Here's how the part is built. I have some questions about the finished solid (model axes, mm). A direction names the side the tool comes from. Round coordinates to 2 decimals unless told otherwise and drop trailing zeros. Write each loop counter-clockwise with the first axis right and the second up, starting at its lowest first coordinate (ties: lowest second). Pieces come first, ordered by that corner, then holes. Notation, with made-up numbers: (87.25, -5.75) -> (142.25, -5.75) arc R17 ccw to (142.25, 10.25) -> close; hole circle Ø11 at (2.5, 66.25). An arc over 180 degrees is marked (long way). Put each result on its own line as item: value. Start each with the question number.
1) Will these pins go through, and if not, where does the flat tip stop? P1, Ø18.5, axis at x = 944, y = 37, coming from the -Z side (3 decimals); P2, Ø8, axis at x = 1001.5, y = -37, coming from the -Z side (3 decimals); P3, Ø16, axis at y = -16.5, z = 1330, coming from the -X side.
2) I want a section at A-A, the plane z = 1916.5. Give the number of separate pieces and of enclosed holes in the cut face, then the cut area to 3 significant figures.
3) If I drill on line 1 along X through (y, z) = (21.5, 1035.5) (3 decimals); line 2 along X through (y, z) = (-31, 1517) (3 decimals); line 3 along Z through (x, y) = (233, 15.5) (3 decimals), over which ranges is the centre line in solid material (lowest first)? Write a range as [from, to].
4) We'd pull the mould along X, two halves only. Please class faces 1 (the flat face through (28, 3.175, 1032)), 2 (the flat face through (25, 65.088, 1041)), 3 (the flat face through (1570.831, 6, 1022)), 4 (the flat face through (31.75, 34, 1006)): released by +X, released by -X, zero draft, split by the parting line, or undercut.
5) I want a section at B-B, the plane x = 1331.5. List the corners of the cut face in (y, z) for me (1 decimal).
6) Which directions (+Z, -Z, +X, -X, +Y, -Y) give clear straight access to the entire face, cutting with the end or side of a thin tool? Please do faces 5 (the flat face through (607, -50.8, 1041)), 6 (the flat face through (1086, 34, 2041.525)), 7 (the flat face through (1085, -23, 2054.225)).
from build123d import *

# Parameters (mm, degrees)
F3_DEPTH      = 61.9125
F5_DEPTH      = 50.8
F5_DEPTH_BACK = 3.175


with BuildPart() as f3:
    # F2 (on offset) → F3 (new body)
    with BuildSketch(Plane.XZ.offset(-3.175)):
        Polygon((0, 2054.225), (0, 0), (19.05, 0), (31.75, 0), (31.75, 2041.525), (581.025, 2041.525), (581.025, 0), (593.725, 0), (612.775, 0), (631.825, 0), (644.525, 0), (644.525, 2041.525), (1539.08125, 2041.525), (1539.08125, 0), (1551.78125, 0), (1570.83125, 0), (1570.83125, 2073.275), (0, 2073.275), align=None)
    extrude(amount=-F3_DEPTH)

    # F4 (on Front) → F5 (join, two sides)
    with BuildSketch(Plane.XZ) as f5_sk:
        Polygon((0, 2054.225), (0, 0), (19.05, 0), (19.05, 2041.525), (19.05, 2054.225), (593.725, 2054.225), (593.725, 0), (612.775, 0), (631.825, 0), (631.825, 2054.225), (1551.78125, 2054.225), (1551.78125, 2041.525), (1551.78125, 0), (1570.83125, 0), (1570.83125, 2073.275), (0, 2073.275), align=None)
    extrude(amount=F5_DEPTH)
    extrude(f5_sk.sketch, amount=-F5_DEPTH_BACK)


solid = f3.part
Findings:
1. P1: stops at z = 2041.525
1. P2: stops at z = 2054.225
1. P3: stops at x = 0
2. separate pieces: 3
2. enclosed holes: 0
2. area: 12,000 mm2
3. line 1: x = [0, 31.75], [581.025, 644.525], [1539.081, 1570.831]
3. line 2: x = [0, 19.05], [593.725, 631.825], [1551.781, 1570.831]
3. line 3: z = [2041.525, 2073.275]
4. face 1: undercut
4. face 2: zero draft
4. face 3: released by +X
4. face 4: undercut
5. outline: (-50.8, 2054.2) -> (3.2, 2054.2) -> (3.2, 2041.5) -> (65.1, 2041.5) -> (65.1, 2073.3) -> (-50.8, 2073.3) -> close
6. face 5: +Z, -Z, +X, -X, -Y
6. face 6: -Z, +Y, -Y
6. face 7: -Z, -Y
